```python
from build123d import *

# Parameters (mm, degrees)
SKETCH1_W           = 23
SKETCH1_H           = 15
SKETCH1_W_2         = 19
SKETCH1_H_2         = 12
BOSS_EXTRUDE1_DEPTH = 35
CHAMFER1_SIZE       = 1
CHAMFER2_SIZE       = 1
SKETCH2_W           = 23
SKETCH2_H           = 15
BOSS_EXTRUDE2_DEPTH = 3
CHAMFER4_SIZE       = 1.5
SKETCH3_R           = 2.5
CUT_EXTRUDE1_DEPTH  = 3
SKETCH5_R           = 6.5
CUT_EXTRUDE3_DEPTH  = 40


with BuildPart() as part:
    # Sketch1 → Boss-Extrude1 (new body)
    with BuildSketch(Plane(origin=(0, 0, 0), x_dir=(1, 0, 0), z_dir=(0, 1, 0))):
        Rectangle(SKETCH1_W, SKETCH1_H)
        Rectangle(SKETCH1_W_2, SKETCH1_H_2, mode=Mode.SUBTRACT)
    extrude(amount=BOSS_EXTRUDE1_DEPTH)

    # Chamfer1
    chamfer1_edges = [part.edges().sort_by_distance(p)[0] for p in [
        (-11.5, 35, 0),
        (0, 35, 7.5),
        (11.5, 35, 0),
        (0, 35, -7.5),
    ]]
    chamfer(chamfer1_edges, length=CHAMFER1_SIZE)

    # Chamfer2
    chamfer2_edges = [part.edges().sort_by_distance(p)[0] for p in [
        (9.5, 17.5, 6),
        (9.5, 17.5, -6),
        (-9.5, 17.5, -6),
        (-9.5, 17.5, 6),
    ]]
    chamfer(chamfer2_edges, length=CHAMFER2_SIZE)

    # Sketch2 → Boss-Extrude2 (add)
    with BuildSketch(Plane.XZ):
        Rectangle(SKETCH2_W, SKETCH2_H)
    extrude(amount=BOSS_EXTRUDE2_DEPTH)

    # Chamfer4
    chamfer4_edges = [part.edges().sort_by_distance(p)[0] for p in [
        (-11.5, 15.5, 7.5),
        (-11.5, 15.5, -7.5),
        (11.5, 15.5, -7.5),
        (11.5, 15.5, 7.5),
    ]]
    chamfer(chamfer4_edges, length=CHAMFER4_SIZE)

    # Sketch3 → Cut-Extrude1 (cut)
    with BuildSketch(Plane.XZ.offset(3)):
        with Locations(Location((0, 0, 0), (0, 0, 270))):
            Circle(SKETCH3_R)
    extrude(amount=-CUT_EXTRUDE1_DEPTH, mode=Mode.SUBTRACT)

    # Sketch5 → Cut-Extrude3 (cut)
    with BuildSketch(Plane(origin=(0, 0, 0), x_dir=(1, 0, 0), z_dir=(0, 1, 0))):
        Circle(SKETCH5_R)
    extrude(amount=CUT_EXTRUDE3_DEPTH, mode=Mode.SUBTRACT)


solid = part.part
```
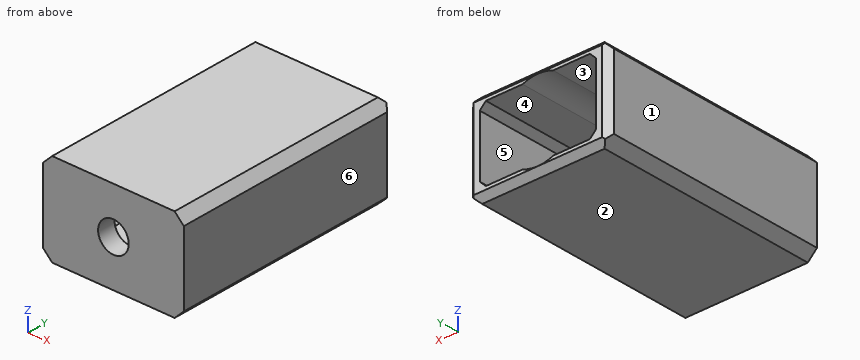
Geometry: final body of the model. Coordinates: model frame, mm. Face numbers are marked on the shaded views. A direction names the side the tool comes from. Round coordinates to 2 decimals unless told otherwise and drop trailing zeros. Order: outer loops, then holes, each group sorted by start corner. A loop starts at its lowest first (then second) coordinate and runs counter-clockwise, first axis right, second up. Notation, with made-up numbers: M 76,-28.75 L 123,-28.75 A25 cw 123,-3.75 Z; hole C 39,41 d3. An arc over 180 degrees is marked long. Use one line per item in the form item = value. Start each with the question number.
Q1. Access query for the marked faces 5 and 6. Directions: +Z, -Z, +X, -X, +Y, -Y. A direction counts if a zero-diameter tool reaches every point of the face in a straight line with its end or side. Return the directions, or none.
Q2. Cut plane D-D (x = -7). Return loops of the section in (y, z).
Q3. Cut plane A-A (z = 0). Return loops of the section in (x, y), and give its area (3 significant figures).
Q4. Material intervals for line 1 (X direction, y = 13, z = 1.25); line 2 (Z direction, x = -7.75, y = 26); line 3 (X direction, y = -2.1, z = 0), sorted ascending. Write a range as [from, to].
Q5. Cut plane C-C (z = -5.5). Return loops of the section in (x, y), and give its area (3 significant figures).
Q6. Mould query, pull axis Z, two halves, no side actions, for the marked faces 1, 2, 3 and 4. Classes: +Z half, -Z half, draft (parallel to the pull), parting line (faces both ways), or undercut.
Q7. Cut plane B-B (y = 19). Return loops of the section in (x, z).
Q8. Pin query (flat end, axial travel): pin 1 Ø4 at (x, z) = (-7.5, -4.5) entering from +Y; pin 2 Ø1 at (x, z) = (1, 5.5) entering from +Y. Return the tip coordinate at first contact, or that it passes through.
Geometry results:
q1.face_5 = +Y
q1.face_6 = +Z, -Z, +X, +Y, -Y
q2.outline = M -3,-7.5 L 34,-7.5 L 35,-6.5 L 35,-6 L 0,-6 L 0,6 L 35,6 L 35,6.5 L 34,7.5 L -3,7.5 Z
q3.outline = M -11.5,-3 L -2.5,-3 L -2.5,0 L -9.5,0 L -9.5,35 L -10.5,35 L -11.5,34 Z; M 2.5,-3 L 11.5,-3 L 11.5,34 L 10.5,35 L 9.5,35 L 9.5,0 L 2.5,0 Z
q3.area = 193 mm^2
q4.line_1 = [-11.5, -9.5], [9.5, 11.5]
q4.line_2 = [-7.5, -6], [6, 7.5]
q4.line_3 = [-11.5, -2.5], [2.5, 11.5]
q5.outline = M -11.5,-3 L 11.5,-3 L 11.5,34 L 10.5,35 L 9,35 L 9,0 L -9,0 L -9,35 L -10.5,35 L -11.5,34 Z
q5.area = 243 mm^2
q6.face_1 = draft
q6.face_2 = -Z half
q6.face_3 = undercut
q6.face_4 = undercut
q7.outline = M -11.5,-6 L -10,-7.5 L 10,-7.5 L 11.5,-6 L 11.5,6 L 10,7.5 L -10,7.5 L -11.5,6 Z; hole M -9.5,-5 L -8.5,-6 L -2.5,-6 A6.5 ccw 2.5,-6 L 8.5,-6 L 9.5,-5 L 9.5,5 L 8.5,6 L 2.5,6 A6.5 ccw -2.5,6 L -8.5,6 L -9.5,5 Z
q8.pin_1 = 35
q8.pin_2 = 0
